```python
from build123d import *

# Parameters (mm, degrees)
SKETCH1_R                = 5.11
SKETCH1_R_2              = 3.97
BOSS_EXTRUDE1_DEPTH      = 0.5
SKETCH2_R                = 0.6
BOSS_EXTRUDE2_DEPTH      = 0.5
FILLET1_R                = 0.3
SKETCH5_R                = 0.3
CUT_EXTRUDE1_DEPTH       = 0.2
CIRPATTERN4_COUNT        = 8
FILLET1_OF_CIRPATTERN4_R = 0.3
FILLET2_R                = 0.3
FILLET3_R                = 0.3


with BuildPart() as part:
    # Sketch1 → Boss-Extrude1 (new body)
    with BuildSketch(Plane(origin=(0, 0, 0), x_dir=(1, 0, 0), z_dir=(0, 1, 0))):
        with Locations(Location((0, 0, 0), (0, 0, 270))):
            Circle(SKETCH1_R)
        with Locations(Location((0, 0, 0), (0, 0, 270))):
            Circle(SKETCH1_R_2, mode=Mode.SUBTRACT)
    extrude(amount=BOSS_EXTRUDE1_DEPTH)

    # Sketch2 → Boss-Extrude2 (add)
    with BuildSketch(Plane(origin=(0, 0.5, 0), x_dir=(1, 0, 0), z_dir=(0, 1, 0))):
        with Locations((0, 3.97)):
            Circle(SKETCH2_R)
    boss_extrude2 = extrude(amount=-BOSS_EXTRUDE2_DEPTH)

    # Fillet1
    fillet1_edges = [part.edges().sort_by_distance(p)[0] for p in [
        (-0.598284447, 0.25, -3.92465995),
        (0.598284447, 0.25, -3.92465995),
    ]]
    fillet(fillet1_edges, radius=FILLET1_R)

    # Sketch5 → Cut-Extrude1 (cut)
    with BuildSketch(Plane(origin=(0, 0.5, 0), x_dir=(1, 0, 0), z_dir=(0, 1, 0))):
        with Locations(Location((0, 3.97, 0), (0, 0, 270))):
            Circle(SKETCH5_R)
    cut_extrude1 = extrude(amount=-CUT_EXTRUDE1_DEPTH, mode=Mode.SUBTRACT)

    # CirPattern4: Boss-Extrude2, Cut-Extrude1 ×8 about axis
    cirpattern4_axis = Axis((0, 0, 0), (0, 1, 0))
    add([boss_extrude2.rotate(cirpattern4_axis, i * 360 / CIRPATTERN4_COUNT) for i in range(1, CIRPATTERN4_COUNT)])
    add([cut_extrude1.rotate(cirpattern4_axis, i * 360 / CIRPATTERN4_COUNT) for i in range(1, CIRPATTERN4_COUNT)], mode=Mode.SUBTRACT)

    # Fillet1 of CirPattern4
    fillet1_of_cirpattern4_edges = [part.edges().sort_by_distance(p)[0] for p in [
        (-3.198204654, 0.25, -2.352102674),
        (-2.352102674, 0.25, -3.198204654),
        (-3.92465995, 0.25, 0.598284447),
        (-3.92465995, 0.25, -0.598284447),
        (-2.352102674, 0.25, 3.198204654),
        (-3.198204654, 0.25, 2.352102674),
        (0.598284447, 0.25, 3.92465995),
        (-0.598284447, 0.25, 3.92465995),
        (3.198204654, 0.25, 2.352102674),
        (2.352102674, 0.25, 3.198204654),
        (3.92465995, 0.25, -0.598284447),
        (3.92465995, 0.25, 0.598284447),
        (2.352102674, 0.25, -3.198204654),
        (3.198204654, 0.25, -2.352102674),
    ]]
    fillet(fillet1_of_cirpattern4_edges, radius=FILLET1_OF_CIRPATTERN4_R)

    # Fillet2
    # the kernel refuses this fillet: 0.3 mm, written as the material it adds along each edge
    with BuildSketch(Plane(origin=(-2.807213921, 0.3, -2.807213921), x_dir=(0.7071067811865475, 0, 0.7071067811865475), z_dir=(-0.7071067811865475, 0, 0.7071067811865475))) as fillet2_piece_1:
        with BuildLine():
            CenterArc((0.017157288, 0.3), FILLET2_R, 270, 70.528779366)
            Line((0.017157288, 0), (0.017157288, -0.006))
            Line((0.017157288, -0.006), (0.3, -0.006))
            Line((0.3, -0.006), (0.306, 0))
            ThreePointArc((0.306, 0), (0.306, 0.1), (0.305656854, 0.198))
            Line((0.305656854, 0.198), (0.3, 0.2))
        make_face()
    revolve(axis=Axis((-2.807213921, 0.3, -2.807213921), (0, 1, 0)))
    with BuildSketch(Plane(origin=(-3.97, 0.3, 0), x_dir=(1, 0, 0), z_dir=(0, 0, 1))) as fillet2_piece_2:
        with BuildLine():
            CenterArc((0.017157288, 0.3), FILLET2_R, 270, 70.528779366)
            Line((0.017157288, 0), (0.017157288, -0.006))
            Line((0.017157288, -0.006), (0.3, -0.006))
            Line((0.3, -0.006), (0.306, 0))
            ThreePointArc((0.306, 0), (0.306, 0.1), (0.305656854, 0.198))
            Line((0.305656854, 0.198), (0.3, 0.2))
        make_face()
    revolve(axis=Axis((-3.97, 0.3, 0), (0, 1, 0)))
    with BuildSketch(Plane(origin=(-2.807213921, 0.3, 2.807213921), x_dir=(0.7071067811865475, 0, -0.7071067811865475), z_dir=(0.7071067811865475, 0, 0.7071067811865475))) as fillet2_piece_3:
        with BuildLine():
            CenterArc((0.017157288, 0.3), FILLET2_R, 270, 70.528779366)
            Line((0.017157288, 0), (0.017157288, -0.006))
            Line((0.017157288, -0.006), (0.3, -0.006))
            Line((0.3, -0.006), (0.306, 0))
            ThreePointArc((0.306, 0), (0.306, 0.1), (0.305656854, 0.198))
            Line((0.305656854, 0.198), (0.3, 0.2))
        make_face()
    revolve(axis=Axis((-2.807213921, 0.3, 2.807213921), (0, 1, 0)))
    with BuildSketch(Plane(origin=(0, 0.3, 3.97), x_dir=(0, 0, -1), z_dir=(1, 0, 0))) as fillet2_piece_4:
        with BuildLine():
            CenterArc((0.017157288, 0.3), FILLET2_R, 270, 70.528779366)
            Line((0.017157288, 0), (0.017157288, -0.006))
            Line((0.017157288, -0.006), (0.3, -0.006))
            Line((0.3, -0.006), (0.306, 0))
            ThreePointArc((0.306, 0), (0.306, 0.1), (0.305656854, 0.198))
            Line((0.305656854, 0.198), (0.3, 0.2))
        make_face()
    revolve(axis=Axis((0, 0.3, 3.97), (0, 1, 0)))
    with BuildSketch(Plane(origin=(2.807213921, 0.3, 2.807213921), x_dir=(-0.7071067811865475, 0, -0.7071067811865475), z_dir=(0.7071067811865475, 0, -0.7071067811865475))) as fillet2_piece_5:
        with BuildLine():
            CenterArc((0.017157288, 0.3), FILLET2_R, 270, 70.528779366)
            Line((0.017157288, 0), (0.017157288, -0.006))
            Line((0.017157288, -0.006), (0.3, -0.006))
            Line((0.3, -0.006), (0.306, 0))
            ThreePointArc((0.306, 0), (0.306, 0.1), (0.305656854, 0.198))
            Line((0.305656854, 0.198), (0.3, 0.2))
        make_face()
    revolve(axis=Axis((2.807213921, 0.3, 2.807213921), (0, 1, 0)))
    with BuildSketch(Plane(origin=(3.97, 0.3, 0), x_dir=(-1, 0, 0), z_dir=(0, 0, -1))) as fillet2_piece_6:
        with BuildLine():
            CenterArc((0.017157288, 0.3), FILLET2_R, 270, 70.528779366)
            Line((0.017157288, 0), (0.017157288, -0.006))
            Line((0.017157288, -0.006), (0.3, -0.006))
            Line((0.3, -0.006), (0.306, 0))
            ThreePointArc((0.306, 0), (0.306, 0.1), (0.305656854, 0.198))
            Line((0.305656854, 0.198), (0.3, 0.2))
        make_face()
    revolve(axis=Axis((3.97, 0.3, 0), (0, 1, 0)))
    with BuildSketch(Plane(origin=(2.807213921, 0.3, -2.807213921), x_dir=(-0.7071067811865475, 0, 0.7071067811865475), z_dir=(-0.7071067811865475, 0, -0.7071067811865475))) as fillet2_piece_7:
        with BuildLine():
            CenterArc((0.017157288, 0.3), FILLET2_R, 270, 70.528779366)
            Line((0.017157288, 0), (0.017157288, -0.006))
            Line((0.017157288, -0.006), (0.3, -0.006))
            Line((0.3, -0.006), (0.306, 0))
            ThreePointArc((0.306, 0), (0.306, 0.1), (0.305656854, 0.198))
            Line((0.305656854, 0.198), (0.3, 0.2))
        make_face()
    revolve(axis=Axis((2.807213921, 0.3, -2.807213921), (0, 1, 0)))
    with BuildSketch(Plane(origin=(0, 0.3, -3.97), x_dir=(0, 0, 1), z_dir=(-1, 0, 0))) as fillet2_piece_8:
        with BuildLine():
            CenterArc((0.017157288, 0.3), FILLET2_R, 270, 70.528779366)
            Line((0.017157288, 0), (0.017157288, -0.006))
            Line((0.017157288, -0.006), (0.3, -0.006))
            Line((0.3, -0.006), (0.306, 0))
            ThreePointArc((0.306, 0), (0.306, 0.1), (0.305656854, 0.198))
            Line((0.305656854, 0.198), (0.3, 0.2))
        make_face()
    revolve(axis=Axis((0, 0.3, -3.97), (0, 1, 0)))

    # Fillet3
    fillet3_edges = [part.edges().sort_by_distance(p)[0] for p in [
        (-3.019345956, 0.5, -3.019345956),
        (-4.27, 0.5, 0),
        (-3.019345956, 0.5, 3.019345956),
        (0, 0.5, 4.27),
        (3.019345956, 0.5, 3.019345956),
        (4.27, 0.5, 0),
        (3.019345956, 0.5, -3.019345956),
        (0, 0.5, -4.27),
    ]]
    fillet(fillet3_edges, radius=FILLET3_R)


solid = part.part
```
Can you work these out from the model? Positions are in its coordinate system, mm. Coordinates: 2 decimals unless noted, no trailing zeros. Loops run counter-clockwise (first coordinate to the right, second up) from the corner with the lowest first, then second, coordinate; pieces in that order, holes last. Notation, with made-up numbers: (-17, 48) -> (30, 48) arc R16 ccw to (30, 73) -> close; hole circle Ø5 at (-13, 35.5). An arc over 180 degrees is marked (long way). Put each result on its own line as item: value. Start each with the question number.
Q1. I want a section at B-B (z = 1). Write out the boundary of the cut face in (x, y), plus the area to 3 significant figures.
Q2. I'm going to push a flat-ended pin straight in: P1, Ø2, axis at x = -1.5, z = 0, coming from the +Y side. Where does the tip first touch, or does it pass through?
Q3. I want a section at A-A (x = -1.5). Write out the boundary of the cut face in (y, z), plus the area to 3 significant figures.
Q4. If I drill on line 1 (X direction, y = 0.1, z = 2); line 2 (Z direction, x = -3.5, y = 0.1); line 3 (Z direction, x = 0.5, y = 0.15), over which ranges is the centre line in solid material (lowest first)? Write a range as [from, to].
Taken from the geometry:
1. outline: (-5.01, 0) -> (-3.84, 0) -> (-3.84, 0.5) -> (-5.01, 0.5) -> close; (3.84, 0) -> (5.01, 0) -> (5.01, 0.5) -> (3.84, 0.5) -> close
1. area: 1.17 mm2
2. P1: passes through
3. outline: (0, -4.88) -> (0.5, -4.88) -> (0.5, -3.68) -> (0, -3.68) -> close; (0, 3.68) -> (0.5, 3.68) -> (0.5, 4.88) -> (0, 4.88) -> close
3. area: 1.21 mm2
4. line 1: x = [-4.7, -3.43], [3.43, 4.7]
4. line 2: z = [-3.72, -1.87], [-0.37, 0.37], [1.87, 3.72]
4. line 3: z = [-5.09, -3.64], [3.64, 5.09]
